For this review, take the finished solid that the model builds, in its own axes (mm). Face numbers are marked on the shaded views. A direction names the side the tool comes from. Coordinates: 2 decimals unless noted, no trailing zeros. Write each loop counter-clockwise with the first axis right and the second up, starting at its lowest first coordinate (ties: lowest second). Pieces come first, ordered by that corner, then holes.
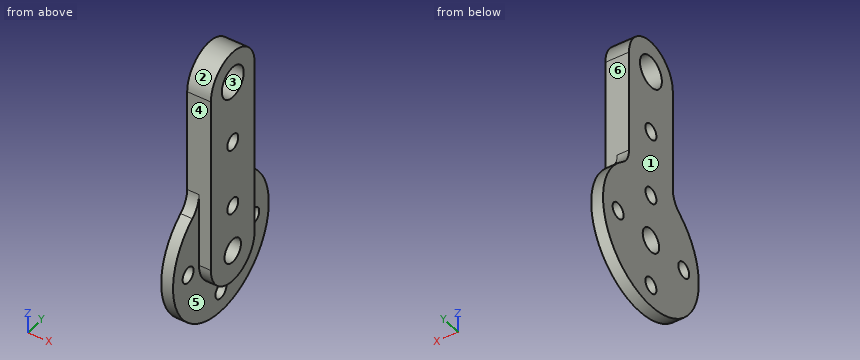
```python
from build123d import *

# Parameters (mm, degrees)
F0_R     = 2
F0_R_2   = 3
F0_R_3   = 4
F1_DEPTH = 6
F2_R     = 2
F3_DEPTH = 6.001
F5_DEPTH = 3


with BuildPart() as f1:
    # F0 (on Right) → F1 (new body)
    with BuildSketch(Plane.YZ):
        with BuildLine():
            ThreePointArc((-8, 18.874586), (-8.640578, 16.177069), (-10.425532, 14.055543))
            ThreePointArc((-10.425532, 14.055543), (0, -17.5), (10.425532, 14.055543))
            ThreePointArc((10.425532, 14.055543), (8.640578, 16.177069), (8, 18.874586))
            Line((8, 18.874586), (8, 45))
            ThreePointArc((8, 45), (0, 53), (-8, 45))
            Line((-8, 45), (-8, 18.874586))
        make_face()
        with Locations((-12, 0)):
            Circle(F0_R, mode=Mode.SUBTRACT)
        with Locations((0, -12)):
            Circle(F0_R, mode=Mode.SUBTRACT)
        Circle(F0_R_2, mode=Mode.SUBTRACT)
        with Locations((0, 12)):
            Circle(F0_R, mode=Mode.SUBTRACT)
        with Locations((12, 0)):
            Circle(F0_R, mode=Mode.SUBTRACT)
        with Locations((0, 45)):
            Circle(F0_R_3, mode=Mode.SUBTRACT)
    extrude(amount=F1_DEPTH)

    # F2 (on face) → F3 (cut, through all)
    with BuildSketch(Plane(origin=(0, 0, 0), x_dir=(0, -1, 0), z_dir=(-1, 0, 0))):
        with Locations((0, 29)):
            Circle(F2_R)
    extrude(amount=-F3_DEPTH, mode=Mode.SUBTRACT)

    # F4 (on face) → F5 (cut)
    with BuildSketch(Plane.YZ.offset(6)):
        with BuildLine():
            Line((-8, 0), (-8, 18.874586))
            ThreePointArc((-8, 18.874586), (0, -20.5), (8, 18.874586))
            Line((8, 18.874586), (8, 0))
            ThreePointArc((8, 0), (0, -8), (-8, 0))
        make_face()
    extrude(amount=-F5_DEPTH, mode=Mode.SUBTRACT)


solid = f1.part
```
Q1. Add section C-C (x = 4.25). State the section outline as (y, z) points.
Ans:
outline: (-8, 0) arc R8 ccw to (8, 0) - (8, 45) arc R8 ccw to (-8, 45) - close; hole circle Ø8 at (0, 45); hole circle Ø6 at (0, 0); hole circle Ø4 at (0, 12); hole circle Ø4 at (0, 29)
Q2. For probe 1 along Z at (x, y) = (3.9, 0); probe 2 along Z at (x, y) = (1.85, 0); probe 3 along Y at (x, z) = (3.35, 8), list the stretches that pass through material, from the lowest coordinate up.
Ans:
probe 1: z = -8 to -3, 3 to 10, 14 to 27, 31 to 41, 49 to 53
probe 2: z = -17.5 to -14, -10 to -3, 3 to 10, 14 to 27, 31 to 41, 49 to 53
probe 3: y = -8 to 8
Q3. Clearance check with flat-ended pins moving along their axes: pin 1 Ø4.5 at (y, z) = (-12, 0) entering from -X; pin 2 Ø4.5 at (y, z) = (0, -12) entering from +X; pin 3 Ø3 at (x, z) = (3, 16) entering from +Y; pin 4 Ø1 at (x, z) = (1.5, 40.5) entering from -Y. State where each tip first meets the part, or that it passes through.
Ans:
pin 1: stops at x = 0
pin 2: stops at x = 3
pin 3: stops at y = 9.89
pin 4: stops at y = -8
Q4. Tool access review of the marked faces 4, 5 and 6: name each direction out of +Z, -Z, +X, -X, +Y, -Y from which nothing blocks a thin tool from reaching the whole face with its end or side.
Ans:
face 4: +Z, +X, -Y
face 5: -Z, +X
face 6: +Z, +X, +Y
Q5. Draft analysis for pull direction Z (two halves, no side actions). For the marked faces 1, 2 and 3, state which applies: +Z half, -Z half, draft (parallel to the pull), parting line (faces both ways), or undercut.
Ans:
face 1: draft
face 2: +Z half
face 3: undercut
Q6. Add section A-A (y = 0). State the section outline as (x, z) points, then the cut area to 4 significant figures.
Ans:
outline: (0, -17.5) - (3, -17.5) - (3, -14) - (0, -14) - close; (0, -10) - (3, -10) - (3, -8) - (6, -8) - (6, -3) - (0, -3) - close; (0, 3) - (6, 3) - (6, 10) - (0, 10) - close; (0, 14) - (6, 14) - (6, 27) - (0, 27) - close; (0, 31) - (6, 31) - (6, 41) - (0, 41) - close; (0, 49) - (6, 49) - (6, 53) - (0, 53) - close
area: 250.5 mm2
Q7. Add section D-D (x = 1.1). State the section outline as (y, z) points, then the cut area to 3 significant figures.
Ans:
outline: (-10.43, 14.06) arc R17.5 ccw (long way) to (10.43, 14.06) arc R6 cw to (8, 18.87) - (8, 45) arc R8 ccw to (-8, 45) - (-8, 18.87) arc R6 cw to start; hole circle Ø4 at (-12, 0); hole circle Ø8 at (0, 45); hole circle Ø6 at (0, 0); hole circle Ø4 at (0, -12); hole circle Ø4 at (0, 12); hole circle Ø4 at (0, 29); hole circle Ø4 at (12, 0)
area: 1,370 mm2
Q8. Add section B-B (z = 29). State the section outline as (x, y) points, then the cut area to 3 significant figures.
Ans:
outline: (0, -8) - (6, -8) - (6, -2) - (0, -2) - close; (0, 2) - (6, 2) - (6, 8) - (0, 8) - close
area: 72.0 mm2
